from build123d import *

# Parameters (mm, degrees)
SKETCH_2_R          = 4.175
EXTRUDE_1_DEPTH     = 5
FILLET_1_R          = 20
SKETCH_6_R          = 0.5000000000000009
CUT_EXTRUDE_3_DEPTH = 47.17452492507412
FILLET_2_R          = 10
CUT_EXTRUDE_4_DEPTH = 57.542041070345505
FILLET_3_R          = 10


with BuildPart() as part:
    # ｽｹｯﾁ2 → ﾎﾞｽ - 押し出し1 (new body)
    with BuildSketch(Plane(origin=(0, 0, 0), x_dir=(1, 0, 0), z_dir=(0, 1, 0))):
        with BuildLine():
            Line((8.269872578160966, 20.67530348178248), (-25.039362549658698, -27.29226699202151))
            Line((-25.039362549658694, -27.292266992021514), (-16.82553632293364, -32.996042821869985))
            Line((-16.82553632293364, -32.996042821869985), (16.77540554807104, 15.391605258271007))
            ThreePointArc((16.775405548070047, 15.39160525826554), (17.036467269075846, 15.346625845237856), (17.298352710232226, 15.306721140237647))
            Line((17.29835271023301, 15.306721140243175), (12.453720459223167, 18.670889747549086))
            ThreePointArc((12.453720459220065, 18.67088974754445), (7.082723548852389, 27.619577165201054), (10.596791286456618, 37.44698487250789))
            Line((10.596791286456803, 37.44698487250808), (9.571486453740173, 38.47228970522472))
            ThreePointArc((9.571486453736274, 38.47228970522862), (5.609855036074267, 29.81593956245965), (8.269872578156503, 20.675303481779164))
        make_face()
        with Locations(Location((-2.3951779892886145, -3.4492196700893225, 0), (0, 0, 270))):
            Circle(SKETCH_2_R, mode=Mode.SUBTRACT)
        with Locations(Location((-16.654617563909806, -23.98378523690196, 0), (0, 0, 270))):
            Circle(SKETCH_2_R, mode=Mode.SUBTRACT)
    extrude_1 = extrude(amount=EXTRUDE_1_DEPTH)

    # ﾌｨﾚｯﾄ1
    # the kernel refuses this fillet: 20 mm, written as the material it adds along each edge
    with BuildSketch(Plane(origin=(16.775405548070545, 0, -15.391605258268275), x_dir=(-0.5703775829850781, 0, 0.8213826226723454), z_dir=(0, 1, 0))) as fillet_1_piece_1_section:
        with BuildLine():
            CenterArc((4.1176832280817175, 20.000000000000004), FILLET_1_R, 257.44880249712094, 12.55119750289515)
            Line((-0.22855499889395509, 0.4779557096502993), (-0.31547976343346945, 0.08751482384330647))
            ThreePointArc((-0.31547976343346945, 0.08751482384330647), (-0.47282168846060246, 0.06752459028858156), (-0.36414407682378114, -0.16552670876373804))
            Line((-0.36414407682378114, -0.16552670876373804), (1.117e-13, -0.3999999999999987))
            Line((1.117e-13, -0.3999999999999987), (4.117683228087442, -0.39999999999999974))
            Line((4.117683228087442, -0.39999999999999974), (4.117683228087329, 1.7e-16))
        make_face()
    fillet_1_piece_1 = extrude(amount=5, mode=Mode.PRIVATE)
    fillet_1_piece_1 = split(fillet_1_piece_1, bisect_by=Plane(origin=(16.82290798810791, 2.5, -15.63687544831251), z_dir=(-0.570377582984848, 0, 0.8213826226725052)), keep=Keep.TOP, mode=Mode.PRIVATE)
    add(fillet_1_piece_1)
    with BuildSketch(Plane(origin=(8.269872578158733, 0, -20.675303481780823), x_dir=(-0.5703775829847766, 0, 0.8213826226725548), z_dir=(0, 1, 0))) as fillet_1_piece_2:
        with BuildLine():
            CenterArc((10.285673470537454, -20.000000000000007), FILLET_1_R, 89.99999999999505, 43.641913313262535)
            Line((-3.5173087138816013, -5.526656128709918), (-3.7933683575699813, -5.237189251284115))
            ThreePointArc((-3.7933683575699813, -5.237189251284115), (-1.7596460761489088, -2.7626969082759216), (-0.3791309613113661, 0.1275135842768152))
            Line((-0.3791309613113661, 0.1275135842768152), (3.413e-14, 0.40000000000000013))
            Line((3.413e-14, 0.40000000000000013), (10.285673470539217, 0.4000000000000006))
            Line((10.285673470539217, 0.4000000000000006), (10.285673470539184, -6e-17))
        make_face()
    extrude(amount=5)

    # ｽｹｯﾁ6 → ｶｯﾄ - 押し出し3 (cut, through all)
    with BuildSketch(Plane(origin=(0, 5, 0), x_dir=(1, 0, 0), z_dir=(0, 1, 0))):
        with Locations(Location((-7.408738509451215, -10.639307664730705, 0), (0, 0, 270))):
            Circle(SKETCH_6_R)
    cut_extrude_3 = extrude(amount=-CUT_EXTRUDE_3_DEPTH, mode=Mode.SUBTRACT)

    # ﾌｨﾚｯﾄ2
    fillet_2_edges = [part.edges().sort_by_distance(p)[0] for p in [
        (17.29835271023262, 2.5, -15.30672114024041),
    ]]
    fillet(fillet_2_edges, radius=FILLET_2_R)

    # ﾐﾗｰ1: ﾎﾞｽ - 押し出し1, ｶｯﾄ - 押し出し3 across plane
    add(extrude_1.mirror(Plane(origin=(4.106913113362459, 5, 2.8518879149242107), x_dir=(-0.5703775829848504, 0, 0.8213826226725034), z_dir=(-0.8213826226725035, 0, -0.5703775829848503))))
    add(cut_extrude_3.mirror(Plane(origin=(4.106913113362459, 5, 2.8518879149242107), x_dir=(-0.5703775829848504, 0, 0.8213826226725034), z_dir=(-0.8213826226725035, 0, -0.5703775829848503))), mode=Mode.SUBTRACT)

    # ｽｹｯﾁ7 → ｶｯﾄ - 押し出し4 (cut, through all)
    with BuildSketch(Plane(origin=(0, 5, 0), x_dir=(1, 0, 0), z_dir=(0, 1, 0))):
        Polygon((-16.825536322933814, -32.99604282186991), (31.619002207822653, 36.767396870690376), (6.63537695599359, 54.116314892564866), (-41.809161574762875, -15.647124799995419), align=None)
    extrude(amount=-CUT_EXTRUDE_4_DEPTH, mode=Mode.SUBTRACT)

    # ﾌｨﾚｯﾄ3
    fillet_3_edges = [part.edges().sort_by_distance(p)[0] for p in [
        (24.69752503161028, 2.5, -9.267751822082793),
        (16.905768195919187, 2.5, -15.579336362687311),
        (21.357815932613555, 2.5, -12.487782977823219),
    ]]
    fillet(fillet_3_edges, radius=FILLET_3_R)


solid = part.part
Can you work these out from the model? Positions are in its coordinate system, mm. Give positions to 0.01 mm unless a question says otherwise; leave off trailing zeros. Loops run counter-clockwise (first coordinate to the right, second up) from the corner with the lowest first, then second, coordinate; pieces in that order, holes last. Notation, with made-up numbers: (-23.5, 83.5) - (23.5, 83.5) arc R26 cw to (23.5, 99.5) - close; hole circle Ø5 at (33, 45.5). An arc over 180 degrees is marked (long way). Return JSON: item names as keys, results as strings.
1. If I drill on line 1 (Z direction, x = 0.5, y = 3.4); line 2 (Z direction, x = -5.5, y = 3.05); line 3 (X direction, y = 1.65, z = 31.5), over which ranges is the centre line in solid material (lowest first)?
Output values:
{"line 1": "z = 8.05 to 15.99, 16.74 to 25.58", "line 2": "z = 16.69 to 26.72, 32.65 to 34.22", "line 3": "x = -15.79 to -12.2, -4.68 to -3.61"}
2. I want a section at D-D on x = -2. Please give me the cut outline in (y, z), and give its area (3 significant figures).
Output values:
{"outline": "(0, 11.65) - (5, 11.65) - (5, 29.18) - (0, 29.18) - close", "area": "87.7 mm²"}
3. I want a section at C-C on y = 1.05. Give the number of separate pieces and of enclosed holes in the cut face, and give its area (3 significant figures).
Output values:
{"separate pieces": "1", "enclosed holes": "3", "area": "495 mm²"}
4. I'm going to push flat-ended pins straight in: pin 1 Ø1.5 at (x, y) = (14, 4) entering from -Z; pin 2 Ø1.5 at (x, y) = (9, 1) entering from +Z; pin 3 Ø3 at (y, z) = (1.5, -2) entering from +X. Where does each tip first touch, or does it pass through?
Output values:
{"pin 1": "stops at z = -10.73", "pin 2": "stops at z = 14.42", "pin 3": "stops at x = 20.69"}
5. I want a section at B-B on x = 8. Please give me the cut outline in (y, z), and give its area (3 significant figures).
Output values:
{"outline": "(0, -2.75) - (5, -2.75) - (5, 5.59) - (0, 5.59) - close; (0, 12.71) - (5, 12.71) - (5, 14.78) - (0, 14.78) - close", "area": "52.1 mm²"}
6. I want a section at A-A on z = 6. Please give me the cut outline in (x, y), and give its area (3 significant figures).
Output values:
{"outline": "(1.92, 0) - (3.08, 0) - (3.08, 5) - (1.92, 5) - close; (8.56, 0) - (14.1, 0) - (14.1, 5) - (8.56, 5) - close", "area": "33.5 mm²"}
7. We'd pull the mould along X, two halves only. Please class faces 1 (the face through (36.225, 2.465, -11.121)), 2 (the face through (-6.54, 2.46, 25.97)), 3 (the face through (-2.887, 2.535, 12.924)): +X half, -X half, draft (parallel to the pull), parting line (faces both ways), or undercut.
Output values:
{"face 1": "+X half", "face 2": "undercut", "face 3": "-X half"}
